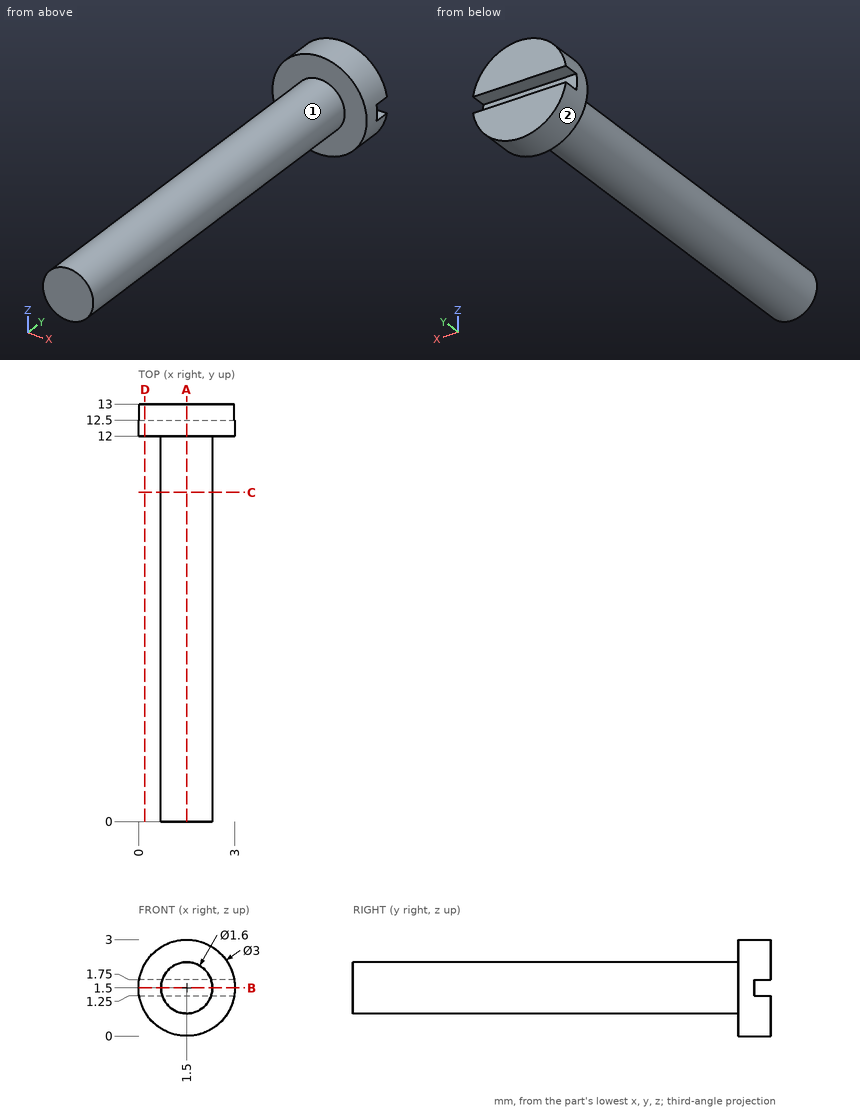
Input: dimensioned drawing with shaded views. Units: mm. Origin: part minimum x, y, z. A direction names the side the tool comes from. Coordinates: 2 decimals unless noted, no trailing zeros. Write each loop counter-clockwise with the first axis right and the second up, starting at its lowest first coordinate (ties: lowest second). Pieces come first, ordered by that corner, then holes. Notation, with made-up numbers: M -37,-9 L 11,-9 A15 cw 11,5 Z; hole C 73,71 d3. An arc over 180 degrees is marked long. Use a Markdown table: item, result.
1) Ray query, L1, parallel to Y at x = 0.65, z = 2.05; L2, parallel to Y at x = 2.5, z = 1.3; L3, parallel to Z at x = 2.7, y = 12.25. Return the intervals inside material, ascending.
Conclusion:
| item | result |
|---|---|
| L1 | y = 12 to 13 |
| L2 | y = 12 to 12.5 |
| L3 | z = 0.6 to 2.4 |
2) Section A-A, the plane x = 1.5. Output: boundary loops of the cut face in (y, z).
Conclusion:
| item | result |
|---|---|
| outline | M 0,0.7 L 12,0.7 L 12,0 L 13,0 L 13,1.25 L 12.5,1.25 L 12.5,1.75 L 13,1.75 L 13,3 L 12,3 L 12,2.3 L 0,2.3 Z |
3) First-contact query: pin 1 Ø1 at (x, z) = (1.5, 1.5) entering from -Y. Flat tip, straight axial feed; report the tip coordinate or a pass-through.
Conclusion:
| item | result |
|---|---|
| pin 1 | stops at y = 0 |
4) Section B-B, the plane z = 1.5. Output: boundary loops of the cut face in (x, y), then the cut area to 3 significant figures.
Conclusion:
| item | result |
|---|---|
| outline | M 0,12 L 0.7,12 L 0.7,0 L 2.3,0 L 2.3,12 L 3,12 L 3,12.5 L 0,12.5 Z |
| area | 20.7 mm^2 |
5) Reachability of the marked faces 1 and 2 from +Z, -Z, +X, -X, +Y, -Y: full face, straight path, thin tool, end or side. Return the list, or none.
Conclusion:
| item | result |
|---|---|
| face 1 | -Y |
| face 2 | +Y, -Y |
6) Section C-C, the plane y = 10.25. Output: boundary loops of the cut face in (x, z), then the cut area to 3 significant figures.
Conclusion:
| item | result |
|---|---|
| outline | C 1.5,1.5 d1.6 |
| area | 2.01 mm^2 |
7) Section D-D, the plane x = 0.2. Output: boundary loops of the cut face in (y, z).
Conclusion:
| item | result |
|---|---|
| outline | M 12,0.75 L 13,0.75 L 13,1.25 L 12.5,1.25 L 12.5,1.75 L 13,1.75 L 13,2.25 L 12,2.25 Z |
